Model file for the job. Use its own axes, mm. Face numbers are marked on the shaded views. A direction names the side the tool comes from. Give positions to 0.01 mm unless a question says otherwise; leave off trailing zeros. Loops run counter-clockwise (first coordinate to the right, second up) from the corner with the lowest first, then second, coordinate; pieces in that order, holes last. Notation, with made-up numbers: M -6.5,61 L 10.5,61 A12 cw 10.5,68 Z; hole C 37.25,52 d7. An arc over 180 degrees is marked long. Answer in a Markdown table with one row per item.
```python
from build123d import *

# Parameters (mm, degrees)
SKETCH1_W            = 64.65
SKETCH1_H            = 41.72
SKETCH1_R            = 1.5
BOSS_EXTRUDE1_DEPTH  = 1.62
SKETCH2_W            = 18
SKETCH2_H            = 15.9
BOSS_EXTRUDE2_DEPTH  = 8.25
FILLET1_R            = 1
FILLET1_OF_MIRROR1_R = 1


with BuildPart() as part:
    # Sketch1 → Boss-Extrude1 (new body)
    with BuildSketch(Plane(origin=(0, 0, 0), x_dir=(1, 0, 0), z_dir=(0, 1, 0))):
        Rectangle(SKETCH1_W, SKETCH1_H)
        with Locations((27.605, -17.61)):
            Circle(SKETCH1_R, mode=Mode.SUBTRACT)
        with Locations((-27.875, -17.61)):
            Circle(SKETCH1_R, mode=Mode.SUBTRACT)
        with Locations((28.875, 17.01)):
            Circle(SKETCH1_R, mode=Mode.SUBTRACT)
        with Locations((-29.325, 17.01)):
            Circle(SKETCH1_R, mode=Mode.SUBTRACT)
    extrude(amount=BOSS_EXTRUDE1_DEPTH)

    # Sketch2 → Boss-Extrude2 (add)
    with BuildSketch(Plane(origin=(0, 1.62, 0), x_dir=(1, 0, 0), z_dir=(0, 1, 0))):
        with Locations((-30.425, 6.11)):
            Rectangle(SKETCH2_W, SKETCH2_H)
    boss_extrude2 = extrude(amount=BOSS_EXTRUDE2_DEPTH)

    # Fillet1
    fillet1_edges = [part.edges().sort_by_distance(p)[0] for p in [
        (-30.425, 9.87, -14.06),
        (-30.425, 9.87, 1.84),
    ]]
    fillet(fillet1_edges, radius=FILLET1_R)

    # Mirror1: Boss-Extrude2 across plane
    add(boss_extrude2.mirror(Plane(origin=(0, 0, 0), x_dir=(0, 0, 1), z_dir=(1, 0, 0))))

    # Fillet1 of Mirror1
    fillet1_of_mirror1_edges = [part.edges().sort_by_distance(p)[0] for p in [
        (30.425, 9.87, -14.06),
        (30.425, 9.87, 1.84),
    ]]
    fillet(fillet1_of_mirror1_edges, radius=FILLET1_OF_MIRROR1_R)


solid = part.part
```
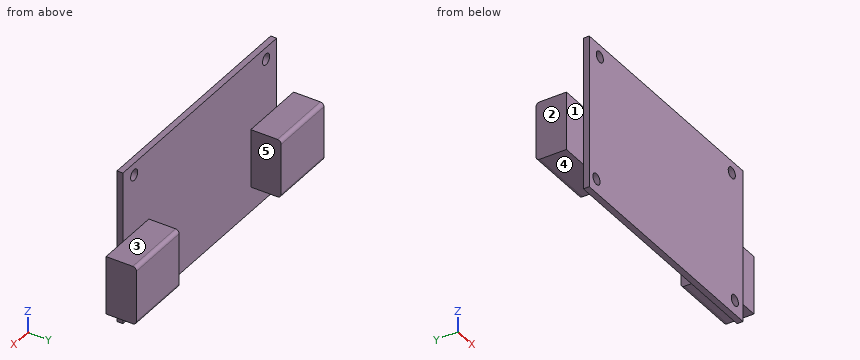
Q1. Saw through at D-D (z = -10). Give the cut face in (x, y) (3 decimals).
Reported:
| item | result |
|---|---|
| outline | M -39.425,1.62 L -32.325,1.62 L -32.325,0 L 32.325,0 L 32.325,1.62 L 39.425,1.62 L 39.425,9.87 L 21.425,9.87 L 21.425,1.62 L -21.425,1.62 L -21.425,9.87 L -39.425,9.87 Z |
Q2. 3-axis set-ups, long thin cutter, end or side, ignore diameter. For the marked faces 1, 2, 3, 4 and 5: which of +Z, -Z, +X, -X, +Y, -Y reach the whole face in a straight line?
Reported:
| item | result |
|---|---|
| face 1 | +Z, -Z, -X, -Y |
| face 2 | +Z, -Z, -X, +Y, -Y |
| face 3 | +Z, +X, -X, +Y |
| face 4 | -Z, +X, -X, +Y |
| face 5 | +Z, -Z, +Y |
Q3. Saw through at C-C (x = 24). Give the cut face in (y, z).
Reported:
| item | result |
|---|---|
| outline | M 0,-20.86 L 1.62,-20.86 L 1.62,-14.06 L 8.87,-14.06 A1 ccw 9.87,-13.06 L 9.87,0.84 A1 ccw 8.87,1.84 L 1.62,1.84 L 1.62,20.86 L 0,20.86 Z |
Q4. Saw through at B-B (y = 8). Give the cut face in (x, z) (3 decimals).
Reported:
| item | result |
|---|---|
| outline | M -39.425,-14.06 L -21.425,-14.06 L -21.425,1.84 L -39.425,1.84 Z; M 21.425,-14.06 L 39.425,-14.06 L 39.425,1.84 L 21.425,1.84 Z |
Q5. Probe probe 1 along X at (y, z) = (1.3, -17.01) (3 decimals); probe 2 along X at (y, z) = (0.55, 17.61) (3 decimals); probe 3 along X at (y, z) = (8, -6.5) (3 decimals). List the from-to ranges inside material, lowest first.
Reported:
| item | result |
|---|---|
| probe 1 | -32.325 to -30.825, -27.825 to 27.375, 30.375 to 32.325 |
| probe 2 | -32.325 to -29.375, -26.375 to 26.105, 29.105 to 32.325 |
| probe 3 | -39.425 to -21.425, 21.425 to 39.425 |
Q6. Saw through at A-A (z = 17.61). Give the cut face in (x, y) (3 decimals).
Reported:
| item | result |
|---|---|
| outline | M -32.325,0 L -29.375,0 L -29.375,1.62 L -32.325,1.62 Z; M -26.375,0 L 26.105,0 L 26.105,1.62 L -26.375,1.62 Z; M 29.105,0 L 32.325,0 L 32.325,1.62 L 29.105,1.62 Z |
Q7. Drop flat-ended pins along their axis: pin 1 (5 mm diameter, centred on y = 4.5, z = 6, fed in from +X); pin 2 (12.5 mm diameter, centred on x = -8.5, z = 2.5, fed in from +Y); pin 3 (2 mm diameter, centred on x = -32, y = 6, fed in from -Z); pin 4 (0.8 mm diameter, centred on y = 1, z = -9, fed in from +X) (3 decimals). Give the stop position or say it passes through.
Reported:
| item | result |
|---|---|
| pin 1 | through |
| pin 2 | y = 1.62 |
| pin 3 | z = -14.06 |
| pin 4 | x = 32.325 |
